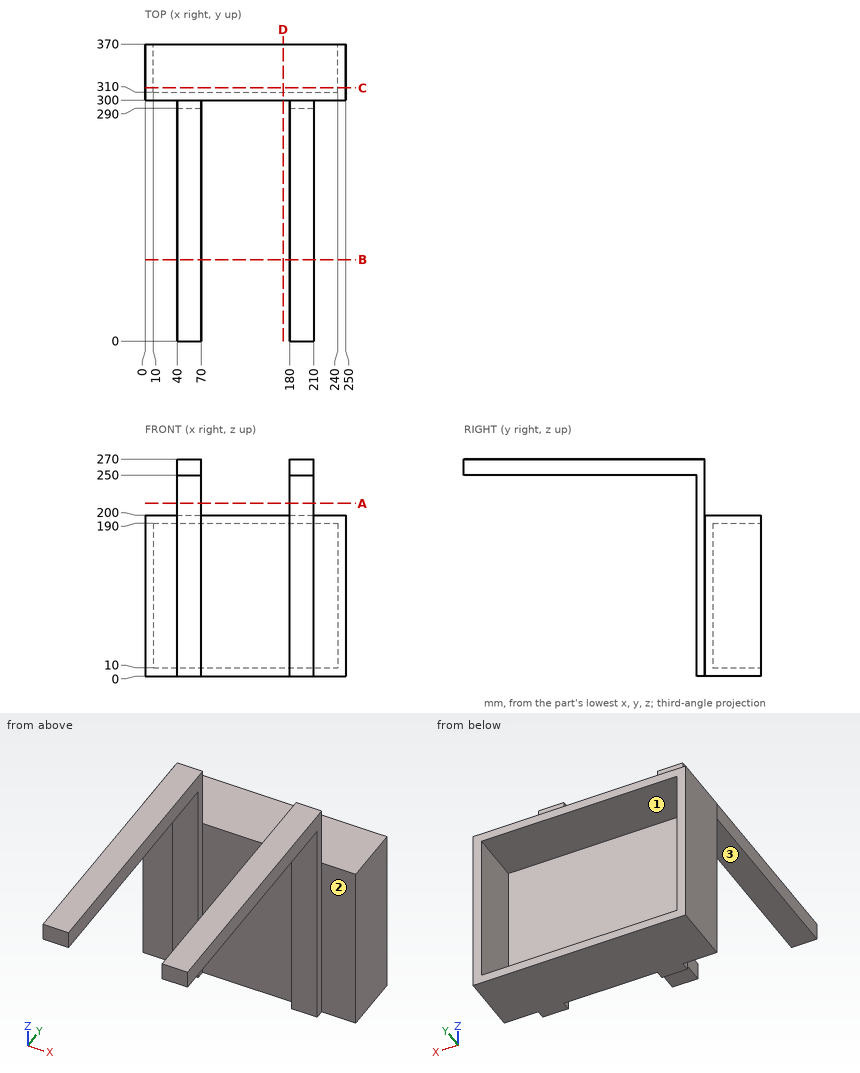
Can you work these out from the drawing? Everything is in mm from the part's minimum corner. A direction names the side the tool comes from. Give positions to 0.01 mm unless a question says otherwise; leave off trailing zeros. Loops run counter-clockwise (first coordinate to the right, second up) from the corner with the lowest first, then second, coordinate; pieces in that order, holes last. Notation, with made-up numbers: (62, 54) -> (101, 54) arc R28 ccw to (101, 82) -> close; hole circle Ø2 at (4, -25). An arc over 180 degrees is marked (long way). Write item = value, one per line.
1) Suppose I cut it at C-C on y = 315.5. Write out the boundary of the cut face in (x, z), then the cut area to 3 significant figures.
Check result:
outline = (0, 0) -> (250, 0) -> (250, 200) -> (0, 200) -> close; hole (10, 10) -> (240, 10) -> (240, 190) -> (10, 190) -> close
area = 8,600 mm2
2) Suppose I cut it at A-A on z = 215. Write out the boundary of the cut face in (x, y), then the cut area to 3 significant figures.
Check result:
outline = (40, 290) -> (70, 290) -> (70, 300) -> (40, 300) -> close; (180, 290) -> (210, 290) -> (210, 300) -> (180, 300) -> close
area = 600 mm2
3) Will these pins go through, and if not, where does the flat tip stop? pin 1 (10 mm diameter, centred on x = 122, z = 147.5, fed in from +Y); pin 2 (12 mm diameter, centred on x = 57.5, z = 124, fed in from -Y); pin 3 (12 mm diameter, centred on x = 239, z = 81.5, fed in from -Y).
Check result:
pin_1 = 310
pin_2 = 290
pin_3 = 300
4) I need wall thicknesses on L1, parallel to Z at x = 237.5, y = 338.5; L2, parallel to X at y = 208, z = 257.5; L3, parallel to X at y = 328.5, z = 169. Which ranges of each line are inside material? Lowest first, please. Write a range as from..to.
Check result:
L1 = 0..10, 190..200
L2 = 40..70, 180..210
L3 = 0..10, 240..250
5) Suppose I cut it at B-B on y = 101.5. Write out the boundary of the cut face in (x, z).
Check result:
outline = (40, 250) -> (70, 250) -> (70, 270) -> (40, 270) -> close; (180, 250) -> (210, 250) -> (210, 270) -> (180, 270) -> close
6) Suppose I cut it at D-D on x = 172. Write out the boundary of the cut face in (y, z).
Check result:
outline = (300, 0) -> (370, 0) -> (370, 10) -> (310, 10) -> (310, 190) -> (370, 190) -> (370, 200) -> (300, 200) -> close
7) For the marked faces 1, 2 and 3, which set-ups out of +Z, -Z, +X, -X, +Y, -Y let a thin tool reach every point of the face, with its end or its side?
Check result:
face_1 = +Y
face_2 = +Z, -Z, +X, -Y
face_3 = -Z, +X, -X, -Y
